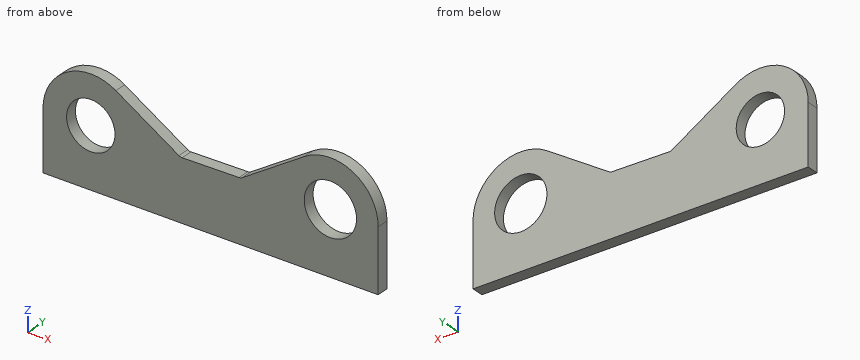
from build123d import *

# Parameters (mm, degrees)
F0_R     = 20.25
F0_R_2   = 21.895042
F1_DEPTH = 10
F2_R     = 5


with BuildPart() as f1:
    # F0 (on Front) → F1 (new body)
    with BuildSketch(Plane.XZ):
        with BuildLine():
            Line((12.9277, 20.534305), (-41.112968, 53.777097))
            ThreePointArc((-41.112968, 53.777097), (-81.586066, 54.623564), (-102.070918, 19.707106))
            Line((-102.070918, 19.707106), (-102.070918, -30.292894))
            Line((-102.070918, -30.292894), (178.429082, -30.292894))
            Line((178.429082, -30.292894), (178.429082, 22.308165))
            ThreePointArc((178.429082, 22.308165), (157.503454, 57.467351), (116.620665, 55.840134))
            Line((116.620665, 55.840134), (63.433077, 21.248158))
            Line((63.433077, 21.248158), (12.9277, 20.534305))
        make_face()
        with Locations((-62.070918, 19.707106)):
            Circle(F0_R, mode=Mode.SUBTRACT)
        with Locations((138.429082, 22.308165)):
            Circle(F0_R_2, mode=Mode.SUBTRACT)
    extrude(amount=F1_DEPTH)

    # F2
    f2_edges = [f1.edges().sort_by_distance(p)[0] for p in [
        (12.9277, -5, 20.534305),
        (63.433077, -5, 21.248158),
    ]]
    fillet(f2_edges, radius=F2_R)


solid = f1.part
Check sheet for the modelled part. Datum: model origin and axes. Units: mm. Round coordinates to 2 decimals unless told otherwise and drop trailing zeros. Loops run counter-clockwise (first coordinate to the right, second up) from the corner with the lowest first, then second, coordinate; pieces in that order, holes last.
1. Sectioned sample at B-B on z = 36.5. Record the boundary of the cut face in (x, y).
2. Sectioned sample at D-D on z = 13.5. Record the boundary of the cut face in (x, y), and give its area (3 significant figures).
3. Gauge pin test, flat ends, axial feed: pin 1 Ø1 at (x, y) = (-55, -5.5) entering from +Z; pin 2 Ø4 at (x, y) = (94.5, -9) entering from +Z; pin 3 Ø2 at (y, z) = (-8, 50) entering from -X. Record the tip position at first contact, or that the pin passes through.
4. Scan lines: probe 1 along X at (y, z) = (-2.25, 38.5); probe 2 along X at (y, z) = (-0.25, 26); probe 3 along X at (y, z) = (-2.75, 17.5). Record each from-to range of solid material in increasing order.
5. Sectioned sample at A-A on y = -8.25. Record the boundary of the cut face in (x, z).
6. Sectioned sample at C-C on x = 153. Record the boundary of the cut face in (y, z).
Recorded:
1. outline: (-98.38, -10) - (-73.39, -10) - (-73.39, 0) - (-98.38, 0) - close; (-50.75, -10) - (-13.03, -10) - (-13.03, 0) - (-50.75, 0) - close; (86.88, -10) - (121.76, -10) - (121.76, 0) - (86.88, 0) - close; (155.1, -10) - (175.83, -10) - (175.83, 0) - (155.1, 0) - close
2. outline: (-102.07, -10) - (-81.35, -10) - (-81.35, 0) - (-102.07, 0) - close; (-42.8, -10) - (118.38, -10) - (118.38, 0) - (-42.8, 0) - close; (158.47, -10) - (178.43, -10) - (178.43, 0) - (158.47, 0) - close
2. area: 2,020 mm2
3. pin 1: stops at z = 59.16
3. pin 2: stops at z = 42.75
3. pin 3: stops at x = -89.31
4. probe 1: x = -97.38 to -69.61, -54.53 to -16.28, 89.96 to 123.69, 153.17 to 175.01
4. probe 2: x = -101.57 to -81.32, -42.82 to 4.04, 70.74 to 116.85, 160.01 to 178.26
4. probe 3: x = -102.07 to -82.2, -41.94 to 117.07, 159.79 to 178.43
5. outline: (-102.07, -30.29) - (178.43, -30.29) - (178.43, 22.31) arc R40 ccw to (116.62, 55.84) - (64.64, 22.04) arc R5 cw to (61.99, 21.23) - (14.38, 20.55) arc R5 cw to (11.69, 21.3) - (-41.11, 53.78) arc R40 ccw to (-102.07, 19.71) - close; hole circle Ø40.5 at (-62.07, 19.71); hole circle Ø43.79 at (138.43, 22.31)
6. outline: (-10, -30.29) - (0, -30.29) - (0, 5.97) - (-10, 5.97) - close; (-10, 38.65) - (0, 38.65) - (0, 59.56) - (-10, 59.56) - close
